```python
from build123d import *

# Parameters (mm, degrees)
F3_R = 2


with BuildPart() as f2:
    # F2: sweep along a path in F1
    with BuildLine(Plane.XY) as f2_path:
        Line((0, 0), (0, 623))
    # F0 (on Front) → F2 (sweep)
    with BuildSketch(Plane.XZ):
        Polygon((40, 0), (0, 0), (0, -350), (27, -350), (27, -376), (29, -376), (29, -348), (2, -348), (2, -2), (38, -2), (38, -25), (40, -25), align=None)
    sweep(path=f2_path.line)

    # F3
    f3_edges = [f2.edges().sort_by_distance(p)[0] for p in [
        (40, 311.5, 0),
        (0, 311.5, 0),
        (29, 311.5, -348),
        (2, 311.5, -348),
        (2, 311.5, -2),
        (38, 311.5, -2),
        (27, 311.5, -350),
        (0, 311.5, -350),
    ]]
    fillet(f3_edges, radius=F3_R)


solid = f2.part
```
Can you work these out from the model? Positions are in its coordinate system, mm. A direction names the side the tool comes from. Coordinates: 2 decimals unless noted, no trailing zeros. Loops run counter-clockwise (first coordinate to the right, second up) from the corner with the lowest first, then second, coordinate; pieces in that order, holes last.
1) Imagine slicing it at A-A on x = 18. List the corners of the cut face in (y, z) for me, plus the area to 3 significant figures.
2) Imagine slicing it at B-B on y = 150. List the corners of the cut face in (x, z) for me, plus the area to 3 significant figures.
3) Which directions (+Z, -Z, +X, -X, +Y, -Y) give clear straight access to the entire face, cutting with the end or side of a thin tool? Please do faces 1 (the flat face through (27, 316, -364)), 2 (the flat face through (0, 316, -173)), 3 (the flat face through (40, 316, -14)), 4 (the flat face through (20, 316, -2)), 5 (the flat face through (16, 316, -348)).
4) Imagine slicing it at C-C on z = -214. List the corners of the cut face in (x, y) for me, plus the area to 3 significant figures.
5) For pin 1 (2 mm diameter, centred on y = 202.5, z = -227, fed in from +X); pin 2 (11.5 mm diameter, centred on x = 16.5, y = 381.5, fed in from -Z); pin 3 (8 mm diameter, centred on y = 211.5, z = -365.5, fed in from +X), each with a flat end and sliding along its axis, tell me the tip position at first contact or that it passes through.
6) I need wall thicknesses on probe 1 along Z at (x, y) = (14, 370.5); probe 2 along X at (y, z) = (139.5, -76.5); probe 3 along X at (y, z) = (333.5, -21). Which ranges of each line are inside material? Lowest first, please.
7) Thinking about a two-plate mould opening in X: for faces 6 (the flat face through (1, 623, -187)), 7 (the flat face through (29, 316, -363)), 8 (the flat face through (38, 316, -14)), which applies, pulls with the +X half, pulls with the -X half, needs draft (parallel to the pull), parting line crosses it, or undercut?
Completed:
1. outline: (0, -350) - (623, -350) - (623, -348) - (0, -348) - close; (0, -2) - (623, -2) - (623, 0) - (0, 0) - close
1. area: 2,490 mm2
2. outline: (0, -348) arc R2 ccw to (2, -350) - (25, -350) arc R2 cw to (27, -352) - (27, -376) - (29, -376) - (29, -350) arc R2 ccw to (27, -348) - (4, -348) arc R2 cw to (2, -346) - (2, -4) arc R2 cw to (4, -2) - (36, -2) arc R2 cw to (38, -4) - (38, -25) - (40, -25) - (40, -2) arc R2 ccw to (38, 0) - (2, 0) arc R2 ccw to (0, -2) - close
2. area: 928 mm2
3. face 1: -Z, -X, +Y, -Y
3. face 2: +Z, -Z, -X, +Y, -Y
3. face 3: +Z, -Z, +X, +Y, -Y
3. face 4: +Y, -Y
3. face 5: +X, +Y, -Y
4. outline: (0, 0) - (2, 0) - (2, 623) - (0, 623) - close
4. area: 1,250 mm2
5. pin 1: stops at x = 2
5. pin 2: stops at z = -350
5. pin 3: stops at x = 29
6. probe 1: z = -350 to -348, -2 to 0
6. probe 2: x = 0 to 2
6. probe 3: x = 0 to 2, 38 to 40
7. face 6: needs draft
7. face 7: pulls with the +X half
7. face 8: undercut
